from build123d import *

# Parameters (mm, degrees)
SKETCH1_R           = 2
SKETCH1_R_2         = 0.75
BOSS_EXTRUDE1_DEPTH = 2
SKETCH2_R           = 4
SKETCH2_R_2         = 3
BOSS_EXTRUDE2_DEPTH = 3


with BuildPart() as part:
    # Sketch1 → Boss-Extrude1 (new body)
    with BuildSketch(Plane(origin=(0, 0, 0), x_dir=(1, 0, 0), z_dir=(0, 1, 0))):
        with BuildLine():
            Line((16.717889357, -2.490486745), (4.852765263, -3.528550595))
            ThreePointArc((4.852765263, -3.528550595), (0, -6), (-4.852765263, -3.528550595))
            Line((-4.852765263, -3.528550595), (-16.717889357, -2.490486745))
            ThreePointArc((-16.717889357, -2.490486745), (-19, 0), (-16.717889357, 2.490486745))
            Line((-16.717889357, 2.490486745), (-4.852765263, 3.528550595))
            ThreePointArc((-4.852765263, 3.528550595), (0, 6), (4.852765263, 3.528550595))
            Line((4.852765263, 3.528550595), (16.717889357, 2.490486745))
            ThreePointArc((16.717889357, 2.490486745), (19, 0), (16.717889357, -2.490486745))
        make_face()
        Circle(SKETCH1_R, mode=Mode.SUBTRACT)
        with Locations((7.5, 0)):
            Circle(SKETCH1_R_2, mode=Mode.SUBTRACT)
        with Locations((10.5, 0)):
            Circle(SKETCH1_R_2, mode=Mode.SUBTRACT)
        with Locations((13.5, 0)):
            Circle(SKETCH1_R_2, mode=Mode.SUBTRACT)
        with Locations((16.5, 0)):
            Circle(SKETCH1_R_2, mode=Mode.SUBTRACT)
        with Locations((-16.5, 0)):
            Circle(SKETCH1_R_2, mode=Mode.SUBTRACT)
        with Locations((-13.5, 0)):
            Circle(SKETCH1_R_2, mode=Mode.SUBTRACT)
        with Locations((-10.5, 0)):
            Circle(SKETCH1_R_2, mode=Mode.SUBTRACT)
        with Locations((-7.5, 0)):
            Circle(SKETCH1_R_2, mode=Mode.SUBTRACT)
    extrude(amount=BOSS_EXTRUDE1_DEPTH)

    # Sketch2 → Boss-Extrude2 (add)
    with BuildSketch(Plane(origin=(0, 2, 0), x_dir=(1, 0, 0), z_dir=(0, 1, 0))):
        Circle(SKETCH2_R)
        Circle(SKETCH2_R_2, mode=Mode.SUBTRACT)
    extrude(amount=BOSS_EXTRUDE2_DEPTH)


solid = part.part
Check sheet for the modelled part. Datum: model origin and axes. Units: mm. A direction names the side the tool comes from. Give positions to 0.01 mm unless a question says otherwise; leave off trailing zeros. Order: outer loops, then holes, each group sorted by start corner. A loop starts at its lowest first (then second) coordinate and runs counter-clockwise, first axis right, second up. Notation, with made-up numbers: M 83,2 L 139,2 A6 cw 139,6 Z; hole C -30.5,-33.75 d6. An arc over 180 degrees is marked long. Answer as CSV lines item,"result". Start each with the question number.
Item 1: Cross-section at B-B on x = 0. Enter the section's corners in (y, z), plus the area to 3 significant figures.
Item 2: Thickness scan on line 1 (X direction, y = 4.2, z = 0); line 2 (Y direction, x = -15.5, z = -1.25); line 3 (Z direction, x = -1, y = 1.9). Record the ranges inside material, lowest first. Write a range as [from, to].
Item 3: Tool access check on faces 5 (the face through (-19, 1, 0)), 6 (the face through (-0.867, 3.479, 3.905)). Record the directions out of +Z, -Z, +X, -X, +Y, -Y that give a thin tool (end or side, any length) a straight path to the whole face; none if there is none.
Item 4: Cross-section at A-A on y = 0.5. State how many separate pieces and enclosed holes the cut face has, plus the area to 3 significant figures.
Item 5: Cross-section at C-C on z = 1.25. Enter the section's corners in (x, y).
Item 6: Cross-section at D-D on y = 4.65. Enter the section's corners in (x, z), plus the area to 3 significant figures.
Item 7: Mould release check, pull along X, two halves, no side actions. Record for faces 1 (the face through (0, 1, 6)), 2 (the face through (19, 1, 0)), 3 (the face through (-11.25, 0.99, -0.03)), 4 (the face through (-1, 2, 2)): +X half, -X half, draft (parallel to the pull), parting line (faces both ways), or undercut.
Item 8: Gauge pin test, flat ends, axial feed: P1, Ø1.7, axis at x = 10.5, z = 0, coming from the +Y side; P2, Ø1.5, axis at y = 3, z = -3, coming from the -X side; P3, Ø1, axis at x = -12.5, y = 0.5, coming from the -Z side. Record the tip position at first contact, or that the pin passes through.
Established:
1,outline,"M 0,-6 L 2,-6 L 2,-4 L 5,-4 L 5,-3 L 2,-3 L 2,-2 L 0,-2 Z; M 0,2 L 2,2 L 2,3 L 5,3 L 5,4 L 2,4 L 2,6 L 0,6 Z"
1,area,"22.0 mm^2"
2,line 1,"x = [-4, -3], [3, 4]"
2,line 2,"y = [0, 2]"
2,line 3,"z = [-5.92, -1.73], [1.73, 5.92]"
3,face 5,"-X, +Y, -Y"
3,face 6,"+Y"
4,separate pieces,"1"
4,enclosed holes,"9"
4,area,"236 mm^2"
5,outline,"M -18.67,0 L -1.56,0 L -1.56,2 L -2.73,2 L -2.73,5 L -3.8,5 L -3.8,2 L -18.67,2 Z; M 1.56,0 L 18.67,0 L 18.67,2 L 3.8,2 L 3.8,5 L 2.73,5 L 2.73,2 L 1.56,2 Z"
6,outline,"C 0,0 d8; hole C 0,0 d6"
6,area,"22.0 mm^2"
7,face 1,"parting line"
7,face 2,"+X half"
7,face 3,"undercut"
7,face 4,"undercut"
8,P1,"stops at y = 2"
8,P2,"stops at x = -3.31"
8,P3,"stops at z = -2.9"
